Input: part model. Units: mm. Frame: model coordinates. A direction names the side the tool comes from. Coordinates: 2 decimals unless noted, no trailing zeros. Write each loop counter-clockwise with the first axis right and the second up, starting at its lowest first coordinate (ties: lowest second). Pieces come first, ordered by that corner, then holes. Notation, with made-up numbers: M 56.5,62.5 L 87.5,62.5 A33 cw 87.5,90.5 Z; hole C -15,74.25 d6. An arc over 180 degrees is marked long. Write each question's results on one line, items separated by ' | '. Start each with the question number.
1. First-contact query: pin 1 (2 mm diameter, centred on x = -4, y = 0.5, fed in from +Z); pin 2 (12 mm diameter, centred on x = -53, z = 18, fed in from -Y); pin 3 (4 mm diameter, centred on y = 2.5, z = 39.5, fed in from +X); pin 4 (2 mm diameter, centred on y = 3.5, z = 59, fed in from -X). Flat tips, straight axial feed; report the tip coordinate or a pass-through.
2. Section query B-B, the plane x = -14. Output: boundary loops of the cut face in (y, z).
3. Section query C-C, the plane z = 49. Output: boundary loops of the cut face in (x, y), and give its area (4 significant figures).
4. Set-up query: faces 4 (the flat face through (-2.111, 0, 67)), 5 (the flat face through (48, 0, 9.065)), 6 (the flat face through (-72.5, 0, 0)), 7 (the flat face through (11, 0, 123.52)), 8 (the flat face through (10.389, 0, -3)). Return all of +Z, -Z, +X, -X, +Y, -Y with unobstructed straight access to the full face (end or side cutting, diameter ignored); none if empty.
5. Ray query, probe 1 along X at (y, z) = (0, 52); probe 2 along Z at (x, y) = (50.5, 5); probe 3 along Z at (x, y) = (14.5, 4). Return the intervals inside material, ascending.
6. Section query A-A, the plane y = 1. Output: boundary loops of the cut face in (x, z), and give its area (3 significant figures).
7. Pull-direction query (Z, two-part tool) for faces 1 (the flat face through (-37, 0, 9.065)), 2 (the flat face through (-1, 0, -9.065)), 3 (the flat face through (15.389, 0, -3)); classes: +Z half, -Z half, draft (parallel to the pull), parting line (faces both ways), or undercut.
```python
from build123d import *

# Parameters (mm, degrees)
F1_DEPTH = 6.25


with BuildPart() as f1:
    # F0 (on Front) → F1 (new body, symmetric)
    with BuildSketch(Plane.XZ):
        Polygon((72.5, -9.064749), (72.5, 9.064749), (22.888701, 9.064749), (22.888701, 123.519985), (-2.111299, 123.519985), (-2.111299, 9.064749), (-72.5, 9.064749), (-72.5, -9.064749), align=None)
        with BuildLine():
            Line((10.388701, 1.997165), (8.559674, 1.997165))
            ThreePointArc((8.559674, 1.997165), (12.888701, 9.723112), (17.217728, 1.997165))
            Line((17.217728, 1.997165), (15.388701, 1.997165))
            Line((15.388701, 1.997165), (15.388701, -8.002835))
            Line((15.388701, -8.002835), (10.388701, -8.002835))
            Line((10.388701, -8.002835), (10.388701, 1.997165))
        make_face(mode=Mode.SUBTRACT)
    extrude(amount=F1_DEPTH, both=True)


solid = f1.part
```
Answer:
1) pin 1: z = 9.06 | pin 2: through | pin 3: x = 22.89 | pin 4: x = -2.11
2) outline: M -6.25,-9.06 L 6.25,-9.06 L 6.25,9.06 L -6.25,9.06 Z
3) outline: M -2.11,-6.25 L 22.89,-6.25 L 22.89,6.25 L -2.11,6.25 Z | area: 312.5 mm^2
4) face 4: +Z, -X, +Y, -Y | face 5: +Z, +X, +Y, -Y | face 6: +Z, -Z, -X, +Y, -Y | face 7: +Z, +X, -X, +Y, -Y | face 8: +Y, -Y
5) probe 1: -2.11 to 22.89 | probe 2: -9.06 to 9.06 | probe 3: -9.06 to -8, 9.46 to 123.52
6) outline: M -72.5,-9.06 L 72.5,-9.06 L 72.5,9.06 L 22.89,9.06 L 22.89,123.52 L -2.11,123.52 L -2.11,9.06 L -72.5,9.06 Z; hole M 8.56,2 L 10.39,2 L 10.39,-8 L 15.39,-8 L 15.39,2 L 17.22,2 A5.08 ccw long Z | area: 5,370 mm^2
7) face 1: +Z half | face 2: -Z half | face 3: undercut
